```python
from build123d import *

# Parameters (mm, degrees)
EXTRUDE_1_DEPTH = 2


with BuildPart() as part:
    # Model → 凸台-拉伸1 (new body)
    with BuildSketch(Plane.XY):
        with BuildLine():
            Line((-97.011702464, 42.464925797), (-144.463489001, 275.476643049))
            ThreePointArc((-144.463489001, 275.476643049), (-153.281496848, 288.227053848), (-167.743625943, 293.810696025))
            Line((-167.743625943, 293.810696025), (-167.745826906, 286.787604353))
            ThreePointArc((-167.745826906, 286.787604353), (-157.689004232, 282.787697452), (-151.354655659, 274.011880359))
            Line((-151.354655659, 274.011880359), (-141.897210514, 227.57115189))
            ThreePointArc((-141.897210514, 227.57115189), (-143.213550528, 224.051355827), (-146.432560896, 222.112364438))
            Line((-146.432560896, 222.112364438), (-138.679952298, 222.112364438))
            Line((-138.679952298, 222.112364438), (-138.679952298, 220.112364438))
            Line((-138.679952298, 220.112364438), (-146.432560896, 220.112364438))
            ThreePointArc((-146.432560896, 220.112364438), (-141.8960614, 218.254319099), (-139.170128432, 214.179831448))
            Line((-139.170128432, 214.179831448), (-127.347591585, 155.11105785))
            ThreePointArc((-127.347591585, 155.11105785), (-128.81680318, 151.936000766), (-131.991729699, 150.466507045))
            Line((-131.991729699, 150.466507045), (-124.202532501, 150.465561187))
            Line((-124.202532501, 150.465561187), (-124.202532501, 148.465561187))
            Line((-124.202532501, 148.465561187), (-131.975142876, 148.465561187))
            ThreePointArc((-131.975142876, 148.465561187), (-127.709998786, 146.718869515), (-124.718064663, 143.213057753))
            Line((-124.718064663, 143.213057753), (-109.314139037, 67.572172034))
            ThreePointArc((-109.314139037, 67.572172034), (-109.945142677, 65.832332797), (-111.744040834, 65.397394195))
            Line((-111.744040834, 65.397394195), (-106.221436179, 57.026239152))
            Line((-106.221436179, 57.026239152), (-107.888289044, 55.920988197))
            Line((-107.888289044, 55.920988197), (-113.250526418, 64.049079845))
            ThreePointArc((-113.250526418, 64.049079845), (-113.869929217, 62.064275394), (-115.91101166, 61.66792833))
            Line((-115.91101166, 61.66792833), (-159.023635769, 86.960168667))
            ThreePointArc((-159.023635769, 86.960168667), (-164.320624855, 91.228378401), (-167.743625943, 97.107049276))
            Line((-167.743625943, 97.107049276), (-167.743625943, 83.960168667))
            Line((-167.743625943, 83.960168667), (-97.011702464, 42.464925797))
        make_face()
    extrude(amount=EXTRUDE_1_DEPTH)


solid = part.part
```
Geometry: final body of the model. Coordinates: model frame, mm. A direction names the side the tool comes from. Coordinates: 2 decimals unless noted, no trailing zeros. Order: outer loops, then holes, each group sorted by start corner. A loop starts at its lowest first (then second) coordinate and runs counter-clockwise, first axis right, second up. Notation, with made-up numbers: (-11, 85) - (37, 85) arc R19 ccw to (37, 102) - close; hole circle Ø5 at (-34.75, -22). An arc over 180 degrees is marked (long way). Return JSON: item names as keys, results as strings. Group by question number.
1. Cut plane A-A (x = -118.5). Output: boundary loops of the cut face in (y, z).
2. Cut plane D-D (y = 163.5). Output: boundary loops of the cut face in (x, z).
3. Pin query (flat end, axial travel): pin 1 (0.6 mm diameter, centred on x = -143, z = 1.5, fed in from -Y); pin 2 (0.6 mm diameter, centred on y = 149.5, z = 1.5, fed in from -X); pin 3 (0.6 mm diameter, centred on x = -130, z = 1.5, fed in from -Y). Return the tip coordinate at first contact, or that it passes through.
4. Set-up query: faces 5 (the face through (-128.782, 151.972, 0.986)), 6 (the face through (-153, 288, 1)), 7 (the face through (-117.124, 105.922, 0.986)). Return all of +Z, -Z, +X, -X, +Y, -Y with unobstructed straight access to the full face (end or side cutting, diameter ignored); none if empty.
5. Cut plane C-C (z = 1.25). Output: boundary loops of the cut face in (x, y) (1 decimal), plus the area to 3 significant figures.
6. Cut plane B-B (y = 75). Output: boundary loops of the cut face in (x, z), plus the area to 3 significant figures.
7. Pull-direction query (Y, two-part tool) for faces 1 (the face through (-132.87, 63.5, 0.99)), 2 (the face through (-127.763, 146.757, 0.986)), 3 (the face through (-120.405, 157.34, 0.986)), 4 (the face through (-127, 159, 0)); classes: pulls with the +Y half, pulls with the -Y half, needs draft (parallel to the pull), parting line crosses it, or undercut.
8. Material intervals for line 1 along Y through (x, z) = (-163, 1.9); line 2 along X through (y, z) = (268.5, 0.5); line 3 along X through (y, z) = (78.5, 1.05), sorted ascending. Write a range as [from, to].
Resolved:
{
 "1": {"outline": "(55.07, 0) - (63.19, 0) - (63.19, 2) - (55.07, 2) - close; (112.68, 0) - (147.98, 0) - (147.98, 2) - (112.68, 2) - close"},
 "2": {"outline": "(-129.03, 0) - (-121.66, 0) - (-121.66, 2) - (-129.03, 2) - close"},
 "3": {"pin 1": "stops at y = 69.27", "pin 2": "stops at x = -124.2", "pin 3": "stops at y = 61.64"},
 "4": {"face 5": "+Z, -Z, -X", "face 6": "+Z, -Z, +X, +Y", "face 7": "+Z, -Z"},
 "5": {"outline": "(-167.7, 84) - (-97, 42.5) - (-144.5, 275.5) arc R26.3 ccw to (-167.7, 293.8) - (-167.7, 286.8) arc R19.3 cw to (-151.4, 274) - (-141.9, 227.6) arc R5.7 cw to (-146.4, 222.1) - (-138.7, 222.1) - (-138.7, 220.1) - (-146.4, 220.1) arc R8.4 cw to (-139.2, 214.2) - (-127.3, 155.1) arc R5.1 cw to (-132, 150.5) - (-124.2, 150.5) - (-124.2, 148.5) - (-132, 148.5) arc R9.8 cw to (-124.7, 143.2) - (-109.3, 67.6) arc R2 cw to (-111.7, 65.4) - (-106.2, 57) - (-107.9, 55.9) - (-113.3, 64) arc R2 cw to (-115.9, 61.7) - (-159, 87) arc R18.7 cw to (-167.7, 97.1) - close", "area": "2,400 mm²"},
 "6": {"outline": "(-152.47, 0) - (-138.64, 0) - (-138.64, 2) - (-152.47, 2) - close; (-110.83, 0) - (-103.64, 0) - (-103.64, 2) - (-110.83, 2) - close", "area": "42.0 mm²"},
 "7": {"face 1": "pulls with the -Y half", "face 2": "undercut", "face 3": "pulls with the +Y half", "face 4": "needs draft"},
 "8": {"line 1": "y = [81.18, 89.84], [285.72, 293.04]", "line 2": "x = [-150.23, -143.04]", "line 3": "x = [-158.44, -144.6], [-111.54, -104.35]"}
}
